Can you work these out from the drawing? Everything is in mm from the part's minimum corner. A direction names the side the tool comes from. Give positions to 0.01 mm unless a question says otherwise; leave off trailing zeros. Write each loop counter-clockwise with the first axis right and the second up, starting at its lowest first coordinate (ties: lowest second). Pieces come first, ordered by that corner, then holes. Notation, with made-up numbers: (28, 46.5) -> (84, 46.5) arc R22 cw to (84, 58.5) -> close; hole circle Ø11 at (29, 41.5). An arc over 180 degrees is marked (long way). Return JSON: item names as keys, results as strings.
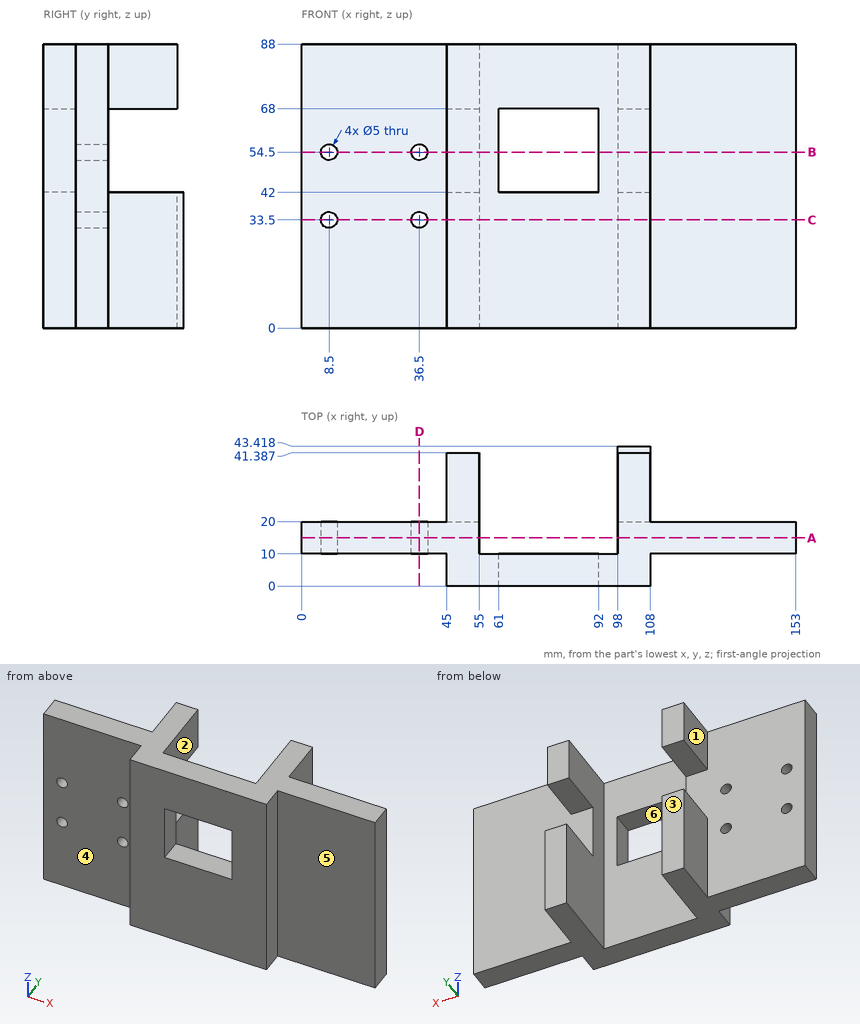
1. Suppose I cut it at B-B, the plane z = 54.5. List the corners of the cut face in (x, y) for me, and give its area (3 significant figures).
Taken from the geometry:
{"outline": "(0, 10) -> (6, 10) -> (6, 20) -> (0, 20) -> close; (11, 10) -> (34, 10) -> (34, 20) -> (11, 20) -> close; (39, 10) -> (45, 10) -> (45, 0) -> (61, 0) -> (61, 10) -> (55, 10) -> (55, 20) -> (39, 20) -> close; (92, 0) -> (108, 0) -> (108, 10) -> (153, 10) -> (153, 20) -> (98, 20) -> (98, 10) -> (92, 10) -> close", "area": "1,320 mm²"}
2. Which directions (+Z, -Z, +X, -X, +Y, -Y) give clear straight access to the entire face, cutting with the end or side of a thin tool? Please do the marked faces 4, 5 and 6.
Taken from the geometry:
{"face 4": "+Z, -Z, -X, -Y", "face 5": "+Z, -Z, +X, -Y", "face 6": "+Y, -Y"}
3. If I drill on line 1 (X direction, y = 16.5, z = 33.5); line 2 (X direction, y = 22, z = 72.5); line 3 (Z direction, x = 8.5, y = 13.5), over which ranges is the centre line in solid material (lowest first)? Write a range as [from, to].
Taken from the geometry:
{"line 1": "x = [0, 6], [11, 34], [39, 55], [98, 153]", "line 2": "x = [45, 55], [98, 108]", "line 3": "z = [0, 31], [36, 52], [57, 88]"}
4. Suppose I cut it at C-C, the plane z = 33.5. List the corners of the cut face in (x, y) for me.
Taken from the geometry:
{"outline": "(0, 10) -> (6, 10) -> (6, 20) -> (0, 20) -> close; (11, 10) -> (34, 10) -> (34, 20) -> (11, 20) -> close; (39, 10) -> (45, 10) -> (45, 0) -> (108, 0) -> (108, 10) -> (153, 10) -> (153, 20) -> (108, 20) -> (108, 43.42) -> (98, 43.42) -> (98, 10) -> (55, 10) -> (55, 41.39) -> (45, 41.39) -> (45, 20) -> (39, 20) -> close"}
5. If we mould it in two halves opening along X, with no side actions, what happens to the marked faces 1, 2 and 3? For each: released by +X, released by -X, zero draft, split by the parting line, or undercut.
Taken from the geometry:
{"face 1": "released by -X", "face 2": "undercut", "face 3": "zero draft"}
6. For pin 1 Ø8 at (y, z) = (4.5, 42.5) entering from +X; pin 2 Ø3 at (x, z) = (36.5, 54.5) entering from -Y; pin 3 Ø3 at (x, z) = (103.5, 74.5) entering from +Y; pin 4 Ø6.5 at (x, z) = (36.5, 33.5) entering from -Y, each with a flat end and sliding along its axis, tell me the tip position at first contact or that it passes through.
Taken from the geometry:
{"pin 1": "stops at x = 108", "pin 2": "passes through", "pin 3": "stops at y = 41.39", "pin 4": "stops at y = 10"}
7. Suppose I cut it at D-D, the plane x = 36.5. List the corners of the cut face in (y, z) for me.
Taken from the geometry:
{"outline": "(10, 0) -> (20, 0) -> (20, 31) -> (10, 31) -> close; (10, 36) -> (20, 36) -> (20, 52) -> (10, 52) -> close; (10, 57) -> (20, 57) -> (20, 88) -> (10, 88) -> close"}
8. Suppose I cut it at A-A, the plane y = 15. List the corners of the cut face in (x, z) for me.
Taken from the geometry:
{"outline": "(0, 0) -> (55, 0) -> (55, 88) -> (0, 88) -> close; (98, 0) -> (153, 0) -> (153, 88) -> (98, 88) -> close; hole circle Ø5 at (8.5, 33.5); hole circle Ø5 at (8.5, 54.5); hole circle Ø5 at (36.5, 33.5); hole circle Ø5 at (36.5, 54.5)"}
